from build123d import *

# Parameters (mm, degrees)
SKETCH2_R           = 100
BOSS_EXTRUDE1_DEPTH = 100
SKETCH3_R           = 90
CUT_EXTRUDE1_DEPTH  = 90
FILLET1_R           = 20
SKETCH4_R           = 4
BOSS_EXTRUDE2_DEPTH = 3


with BuildPart() as part:
    # Sketch2 → Boss-Extrude1 (new body)
    with BuildSketch(Plane(origin=(0, 0, 0), x_dir=(1, 0, 0), z_dir=(0, 1, 0))):
        with Locations(Location((0, 0, 0), (0, 0, 270))):
            Circle(SKETCH2_R)
    extrude(amount=BOSS_EXTRUDE1_DEPTH)

    # Sketch3 → Cut-Extrude1 (cut)
    with BuildSketch(Plane(origin=(0, 100, 0), x_dir=(1, 0, 0), z_dir=(0, 1, 0))):
        with Locations(Location((0, 0, 0), (0, 0, 270))):
            Circle(SKETCH3_R)
    extrude(amount=-CUT_EXTRUDE1_DEPTH, mode=Mode.SUBTRACT)

    # Fillet1
    fillet1_edges = [part.edges().sort_by_distance(p)[0] for p in [
        (0, 0, -100),
    ]]
    fillet(fillet1_edges, radius=FILLET1_R)

    # Sketch4 → Boss-Extrude2 (add)
    with BuildSketch(Plane.XZ):
        with Locations(Location((0, 0, 0), (0, 0, 90))):
            Circle(SKETCH4_R)
    extrude(amount=BOSS_EXTRUDE2_DEPTH)


solid = part.part
Read the model definition and answer for the solid it produces. Units are mm, in the model's axes. A direction names the side the tool comes from. Coordinates: 2 decimals unless noted, no trailing zeros. Order: outer loops, then holes, each group sorted by start corner. A loop starts at its lowest first (then second) coordinate and runs counter-clockwise, first axis right, second up. Notation, with made-up numbers: (32, 23) - (50, 23) arc R10 cw to (50, 30) - close; hole circle Ø4 at (22.5, -20). An arc over 180 degrees is marked (long way). Use one line per item in the form item = value.
(1) Straight lines are drawn through the part: L1, parallel to X at y = 62, z = 0; L2, parallel to Y at x = -52.5, z = 10; L3, parallel to Y at x = 28, z = -76.5. For each, find the intervals that lie inside material, in ascending order.
Computed values:
L1 = -100 to -90, 90 to 100
L2 = 0 to 10
L3 = 0.05 to 10
(2) Section A-A, the plane z = 0 is taken. Give the vertices of the cut face in (x, y).
Computed values:
outline = (-100, 20) arc R20 ccw to (-80, 0) - (-4, 0) - (-4, -3) - (4, -3) - (4, 0) - (80, 0) arc R20 ccw to (100, 20) - (100, 100) - (90, 100) - (90, 10) - (-90, 10) - (-90, 100) - (-100, 100) - close
(3) Given pin 1 Ø1.5 at (x, z) = (-55.5, -80) entering from -Y; pin 2 Ø3 at (x, z) = (-48, 50.5) entering from +Y; pin 3 Ø3 at (x, y) = (70.5, 28.5) entering from +Z; pin 4 Ø4 at (x, y) = (-2, 47) entering from +Z, each flat-ended and moving along its own axis, determine where each tip first touches the part or whether it passes through.
Computed values:
pin_1 = 8.87
pin_2 = 10
pin_3 = 72.38
pin_4 = 100
(4) For a pull along Z with two mould halves and no side action, classify faces 1 (the face through (-34.471, 55.63, 83.137)), 2 (the face through (30.04, 59.44, 95.38)), 3 (the face through (38, 100, -82)) as pulls with the +Z half, pulls with the -Z half, needs draft (parallel to the pull), parting line crosses it, or undercut.
Computed values:
face_1 = undercut
face_2 = parting line crosses it
face_3 = needs draft
(5) Section B-B, the plane x = 0 is taken. Give the vertices of the cut face in (y, z), then the cut area to 3 significant figures.
Computed values:
outline = (-3, -4) - (0, -4) - (0, -80) arc R20 ccw to (20, -100) - (100, -100) - (100, -90) - (10, -90) - (10, 90) - (100, 90) - (100, 100) - (20, 100) arc R20 ccw to (0, 80) - (0, 4) - (-3, 4) - close
area = 3,650 mm²
(6) Which of the six approach directions +Z, -Z, +X, -X, +Y, -Y give full straight-line access (tool end or side, diameter ignored) to faces 4 (the face through (0, -3, 0)), 5 (the face through (1, 10, -1)), 6 (the face through (3.905, -1.479, -0.867))?
Computed values:
face_4 = +Z, -Z, +X, -X, -Y
face_5 = +Y
face_6 = -Y
(7) Section C-C, the plane y = 54.5 is taken. Give the vertices of the cut face in (x, z).
Computed values:
outline = circle Ø200 at (0, 0); hole circle Ø180 at (0, 0)
